from build123d import *

# Parameters (mm, degrees)
SKETCH1_R           = 3.395
BOSS_EXTRUDE1_DEPTH = 124.37
SKETCH3_W           = 6.05
SKETCH3_H           = 0.785
BOSS_EXTRUDE2_DEPTH = 7.98
CUT_EXTRUDE1_DEPTH  = 7.98
SKETCH5_R           = 1.45
CUT_EXTRUDE2_DEPTH  = 7.98


with BuildPart() as part:
    # Sketch1 → Boss-Extrude1 (new body)
    with BuildSketch(Plane(origin=(0, 0, 0), x_dir=(1, 0, 0), z_dir=(0, 1, 0))):
        Circle(SKETCH1_R)
    extrude(amount=BOSS_EXTRUDE1_DEPTH)

    # Sketch3 → Boss-Extrude2 (add)
    with BuildSketch(Plane(origin=(0, 0, 0), x_dir=(1, 0, 0), z_dir=(0, 1, 0))):
        with Locations((0, 0.3925)):
            Rectangle(SKETCH3_W, SKETCH3_H)
        with Locations((0, -0.3925)):
            Rectangle(SKETCH3_W, SKETCH3_H)
    extrude(amount=-BOSS_EXTRUDE2_DEPTH)

    # Sketch4 → Cut-Extrude1 (cut)
    with BuildSketch(Plane(origin=(0, 0, -0.785), x_dir=(-1, 0, 0), z_dir=(0, 0, -1))):
        with BuildLine():
            Line((-3.025, -4.955), (-5.551253647, -4.955))
            Line((-5.551253647, -4.955), (-3.356299124, -8.834088681))
            Line((-3.356299124, -8.834088681), (4.987206478, -9.531994941))
            Line((4.987206478, -9.531994941), (4.886235873, -4.955))
            Line((4.886235873, -4.955), (3.025, -4.955))
            ThreePointArc((3.025, -4.955), (0, -7.98), (-3.025, -4.955))
        make_face()
    extrude(amount=-CUT_EXTRUDE1_DEPTH, mode=Mode.SUBTRACT)

    # Sketch5 → Cut-Extrude2 (cut)
    with BuildSketch(Plane(origin=(0, 0, -0.785), x_dir=(-1, 0, 0), z_dir=(0, 0, -1))):
        with Locations((0, -4.955)):
            Circle(SKETCH5_R)
    extrude(amount=-CUT_EXTRUDE2_DEPTH, mode=Mode.SUBTRACT)


solid = part.part
Here's how the part is built. I have some questions about the finished solid (model axes, mm). A direction names the side the tool comes from. Give positions to 0.01 mm unless a question says otherwise; leave off trailing zeros. Order: outer loops, then holes, each group sorted by start corner. A loop starts at its lowest first (then second) coordinate and runs counter-clockwise, first axis right, second up. Notation, with made-up numbers: (74.25, -1) -> (99.25, -1) arc R26 ccw to (99.25, 24) -> close; hole circle Ø4 at (53, 87). An arc over 180 degrees is marked (long way). Use a Markdown table: item, result. Add a question column.
Item 1: Imagine slicing it at A-A on x = 0. Please give me the cut outline in (y, z) (3 decimals), plus the area to 3 significant figures.
Item 2: Imagine slicing it at B-B on y = 9.5. Please give me the cut outline in (x, z) (3 decimals), plus the area to 3 significant figures.
Item 3: Will these pins go through, and if not, where does the flat tip stop? pin 1 (1 mm diameter, centred on y = 15, z = -2.5, fed in from +X); pin 2 (1 mm diameter, centred on y = 68.5, z = 1, fed in from -X); pin 3 (3 mm diameter, centred on x = -0.5, y = -3, fed in from -Z) (3 decimals).
Item 4: For faces 1 (the face through (0, -3, 0.785)), 2 (the face through (3.24, 61.31, -1.02)), 3 (the face through (0, -3, -0.785)), which set-ups out of +Z, -Z, +X, -X, +Y, -Y let a thin tool reach every point of the face, with its end or its side?
Item 5: I need wall thicknesses on line 1 (Y direction, x = 0.25, z = 0.75); line 2 (X direction, y = 13.5, z = 0.25); line 3 (Y direction, x = -1, z = -2). Which ranges of each line are inside material? Lowest first, please.
Item 6: If we mould it in two halves opening along X, with no side actions, what happens to faces 4 (the face through (0, 124.37, 0)), 5 (the face through (0.189, -3.517, -0.011)), 6 (the face through (-0.07, -7.98, -0.01))? For each: pulls with the +X half, pulls with the -X half, needs draft (parallel to the pull), parting line crosses it, or undercut.
Data:
| question | item | result |
|---|---|---|
| 1 | outline | (-7.98, -0.785) -> (-6.405, -0.785) -> (-6.405, 0.785) -> (-7.98, 0.785) -> close; (-3.505, -0.785) -> (0, -0.785) -> (0, -3.395) -> (124.37, -3.395) -> (124.37, 3.395) -> (0, 3.395) -> (0, 0.785) -> (-3.505, 0.785) -> close |
| 1 | area | 852 mm² |
| 2 | outline | circle Ø6.79 at (0, 0) |
| 2 | area | 36.2 mm² |
| 3 | pin 1 | stops at x = 2.74 |
| 3 | pin 2 | stops at x = -3.36 |
| 3 | pin 3 | stops at z = -0.785 |
| 4 | face 1 | +Z, +X, -X, -Y |
| 4 | face 2 | +Y, -Y |
| 4 | face 3 | -Z, +X, -X, -Y |
| 5 | line 1 | y = -7.97 to -6.38, -3.53 to 124.37 |
| 5 | line 2 | x = -3.39 to 3.39 |
| 5 | line 3 | y = 0 to 124.37 |
| 6 | face 4 | needs draft |
| 6 | face 5 | undercut |
| 6 | face 6 | parting line crosses it |
